from build123d import *

# Parameters (mm, degrees)
CROQUIS2_W              = 20
CROQUIS2_H              = 20
SALIENTE_EXTRUIR1_DEPTH = 8
CROQUIS3_W              = 6.705751287
CROQUIS3_H              = 13
CORTAR_EXTRUIR1_DEPTH   = 6
CORTAR_EXTRUIR2_DEPTH   = 5
CROQUIS6_R              = 1.6
CORTAR_EXTRUIR3_DEPTH   = 3
REDONDEO1_R             = 1


with BuildPart() as part:
    # Croquis2 → Saliente-Extruir1 (new body)
    with BuildSketch(Plane(origin=(0, 0, 0), x_dir=(1, 0, 0), z_dir=(0, 1, 0))):
        with Locations((-0.843373494, -1.526104418)):
            Rectangle(CROQUIS2_W, CROQUIS2_H)
    extrude(amount=SALIENTE_EXTRUIR1_DEPTH)

    # Croquis3 → Cortar-Extruir1 (cut)
    with BuildSketch(Plane(origin=(0, 8, 0), x_dir=(1, 0, 0), z_dir=(0, 1, 0))):
        with Locations((5.803750863, -1.526104418)):
            Rectangle(CROQUIS3_W, CROQUIS3_H)
    extrude(amount=-CORTAR_EXTRUIR1_DEPTH, mode=Mode.SUBTRACT)

    # Croquis5 → Cortar-Extruir2 (cut)
    with BuildSketch(Plane(origin=(0, 8, 0), x_dir=(1, 0, 0), z_dir=(0, 1, 0))):
        with BuildLine():
            Line((2.450875219, -7.526104418), (2.450875219, 4.473895582))
            ThreePointArc((2.450875219, 4.473895582), (2.020425803, 4.459111389), (1.589976387, 4.473895582))
            ThreePointArc((1.589976387, 4.473895582), (-1.703861847, 5.684131739), (-3.832537389, 8.473895582))
            Line((-3.832537389, 8.473895582), (-10.843373494, 8.473895582))
            Line((-10.843373494, 8.473895582), (-10.843373494, -11.526104418))
            Line((-10.843373494, -11.526104418), (-3.832537389, -11.526104418))
            ThreePointArc((-3.832537389, -11.526104418), (-1.703861847, -8.736340574), (1.589976387, -7.526104418))
            ThreePointArc((1.589976387, -7.526104418), (2.020425803, -7.511320225), (2.450875219, -7.526104418))
        make_face()
    extrude(amount=-CORTAR_EXTRUIR2_DEPTH, mode=Mode.SUBTRACT)

    # Croquis6 → Cortar-Extruir3 (cut)
    with BuildSketch(Plane(origin=(0, 3, 0), x_dir=(1, 0, 0), z_dir=(0, 1, 0))):
        with Locations(Location((-7.343373494, -1.526104418, 0), (0, 0, 270))):
            Circle(CROQUIS6_R)
    extrude(amount=-CORTAR_EXTRUIR3_DEPTH, mode=Mode.SUBTRACT)

    # Redondeo1
    redondeo1_edges = [part.edges().sort_by_distance(p)[0] for p in [
        (-10.843373494, 1.5, -8.473895582),
        (-10.843373494, 1.5, 11.526104418),
        (-3.832537389, 5.5, 11.526104418),
        (-3.832537389, 5.5, -8.473895582),
        (9.156626506, 4, -8.473895582),
        (9.156626506, 4, 11.526104418),
    ]]
    fillet(redondeo1_edges, radius=REDONDEO1_R)


solid = part.part
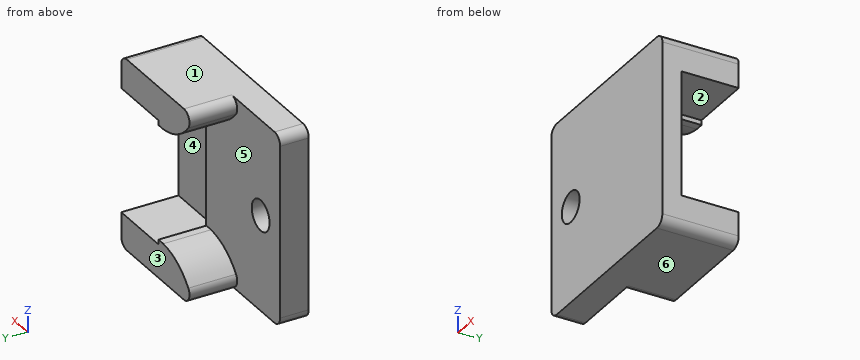
Here's how the part is built. I have some questions about the finished solid (model axes, mm). Face numbers are marked on the shaded views. A direction names the side the tool comes from. Coordinates: 2 decimals unless noted, no trailing zeros. Order: outer loops, then holes, each group sorted by start corner. A loop starts at its lowest first (then second) coordinate and runs counter-clockwise, first axis right, second up. Notation, with made-up numbers: (33, 77) - (86, 77) arc R7 cw to (86, 88) - close; hole circle Ø6 at (9.25, 66.25). An arc over 180 degrees is marked (long way). Use CSV: the item, a comma, the result in double quotes. Start each with the question number.
1. For the marked faces 4, 5 and 6, which set-ups out of +Z, -Z, +X, -X, +Y, -Y let a thin tool reach every point of the face, with its end or its side?
2. Suppose I cut it at D-D on z = 4.5. List the corners of the cut face in (x, y) for me, then the cut area to 3 significant figures.
3. Suppose I cut it at B-B on x = -7. List the corners of the cut face in (y, z) for me.
4. If we mould it in two halves opening along Z, with no side actions, what happens to the marked faces 1, 2 and 3? For each: +Z half, -Z half, draft (parallel to the pull), parting line (faces both ways), or undercut.
5. Suppose I cut it at C-C on z = 2. List the corners of the cut face in (x, y) for me, then the cut area to 3 significant figures.
6. Suppose I cut it at A-A on y = 6.25. List the corners of the cut face in (x, z) for me, then the cut area to 3 significant figures.
7. I'm going to push flat-ended pins straight in: pin 1 (3 mm diameter, centred on x = 6, z = -1.5, fed in from +Y); pin 2 (3 mm diameter, centred on x = -7.34, z = 1.53, fed in from +Y). Where does each tip first touch, or does it pass through?
8. Please list where these lines run through material, in increasing order: line 1 (Z direction, x = 8.25, y = 6); line 2 (Y direction, x = -2.75, z = 6); line 3 (X direction, y = 2.5, z = -4.5). Write a range as from..to.
Output:
1,face 4,"+X, +Y"
1,face 5,"-X, +Y"
1,face 6,"-Z, +X, -X, +Y, -Y"
2,outline,"(-10.84, 0) - (9.16, 0) - (9.16, 2) - (2.45, 2) - (2.45, 3) - (-10.84, 3) - close"
2,area,"53.3 mm2"
3,outline,"(0, -8.47) - (3, -8.47) - (3, -0.04) - (0, -0.04) - close; (0, 3.09) - (3, 3.09) - (3, 11.53) - (0, 11.53) - close"
4,face 1,"+Z half"
4,face 2,"undercut"
4,face 3,"draft"
5,outline,"(-10.84, 0) - (-8.87, 0) - (-8.87, 3) - (-10.84, 3) - close; (-5.82, 0) - (9.16, 0) - (9.16, 2) - (2.45, 2) - (2.45, 3) - (-5.82, 3) - close"
5,area,"44.1 mm2"
6,outline,"(-2.91, -6.86) arc R1 ccw to (-2.13, -8.47) - (8.16, -8.47) arc R1 ccw to (9.16, -7.47) - (9.16, -4.97) - (2.45, -4.97) - (2.45, -4.47) arc R6.27 ccw to start; (-2.91, 9.91) arc R6.27 ccw to (2.45, 7.53) - (2.45, 8.03) - (9.16, 8.03) - (9.16, 10.53) arc R1 ccw to (8.16, 11.53) - (-2.13, 11.53) arc R1 ccw to start"
6,area,"82.6 mm2"
7,pin 1,"stops at y = 2"
7,pin 2,"passes through"
8,line 1,"z = -8.47..-4.97, 8.03..11.52"
8,line 2,"y = 0..3"
8,line 3,"x = -10.84..2.45"
